Autodesk Inventor part; units mm, degrees
ref_plane "YZ Plane" through (0, 0, 0) normal (1, 0, 0) x (0, 1, 0)
ref_plane "XZ Plane" through (0, 0, 0) normal (0, 1, 0) x (-1, 0, 0)
ref_plane "XY Plane" through (0, 0, 0) normal (0, 0, 1) x (1, 0, 0)
sketch "Sketch1" plane through (0, 0, 0) normal (1, 0, 0) x (0, 1, 0)
  line L0 (0, 0) -> (0, -20)
  line L1 (0, -20) -> (8, -20)
  line L2 (8, -20) -> (3, 0)
  line L3 (3, 0) -> (0, 0)
  dimension "d0" = 8
  dimension "d1" = 20
  dimension "d11" = 3
extrude "Extrusion1" add sketch "Sketch1" along normal blind 12
sketch "Sketch2" plane through (0, 0, -20) normal (0, 0, -1) x (-1, 0, 0)
  line L0 (0, 0) -> (0, 8) construction
  line L1 (0, 8) -> (-12, 8) construction
  line L2 (-12, 0) -> (-12, 8) construction
  line L3 (0, 0) -> (-12, 0) construction
  line L4 (-12, 8) -> (0, 0) construction
  line L5 (0, 8) -> (-12, 0) construction
  point P0 (0, 0)
  point P1 (-6, 4)
hole "Hole1" at (6, 4, -20) direction (0, 0, 1) diameter 4.3 depth 7
sketch "Sketch3" plane through (0, 0, 0) normal (-1, 0, 0) x (0, 0, 1)
  line L0 (-20, 0) -> (-20, 8)
  line L1 (-20, 8) -> (0, 3)
  line L2 (0, 3) -> (0, 0)
  line L3 (0, 0) -> (-20, 0)
  line L4 (-20, 15) -> (0, 15)
  line L5 (0, 15) -> (0, 5)
  line L6 (0, 5) -> (-20, 13.9197)
  line L7 (-20, 13.9197) -> (-20, 15)
  dimension "d12" = 15
  dimension "d13" = 2
  dimension "d14" = 10
extrude "Extrusion2" add sketch "Sketch3" against normal up to surface (12 mm away) contours L4 L5 L6 L7
sketch "Sketch4" plane through (0, 0, 0) normal (-1, 0, 0) x (0, 0, 1)
  line L0 (-20, 15) -> (-20, 13.9197)
  line L1 (0, 0) -> (-20, 0)
  line L2 (-20, 15) -> (0, 15)
  line L3 (0, 15) -> (0, 0)
  line L4 (0, 0) -> (-20, 0)
  line L5 (-20, 0) -> (-20, 15)
extrude "Extrusion3" add sketch "Sketch4" along normal blind 2
sketch "Sketch5" plane through (12, 0, 0) normal (1, 0, 0) x (0, 0, -1)
  line L0 (0, 0) -> (0, 15)
  line L1 (0, 15) -> (20, 15)
  line L2 (0, 0) -> (20, 0)
  line L3 (20, 0) -> (20, 15)
  line L4 (20, 15) -> (0, 15)
  line L5 (0, 15) -> (0, 0)
extrude "Extrusion4" add sketch "Sketch5" along normal blind 2
fillet "Fillet1" radius 2 2 edges at (-2, 15, -10) (14, 15, -10)
properties part number "BeltClampNew"
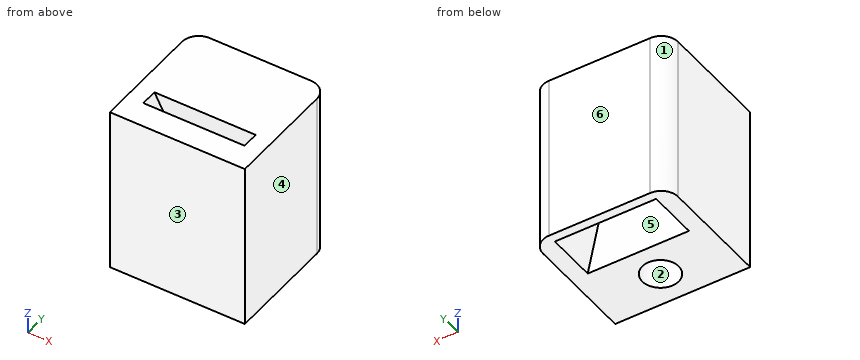
Here's how the part is built. I have some questions about the finished solid (model axes, mm). Face numbers are marked on the shaded views. A direction names the side the tool comes from. Give positions to 0.01 mm unless a question says otherwise; leave off trailing zeros. Loops run counter-clockwise (first coordinate to the right, second up) from the corner with the lowest first, then second, coordinate; pieces in that order, holes last. Notation, with made-up numbers: M 0.5,53.25 L 13.5,53.25 A22 ccw 13.5,89.25 Z; hole C 65.5,28.5 d2. An arc over 180 degrees is marked long. Return JSON: item names as keys, results as strings.
Item 1: Imagine slicing it at A-A on x = 11. List the corners of the cut face in (y, z) for me.
A:
{"outline": "M 0,-20 L 8,-20 L 3,0 L 0,0 Z; M 5,0 L 13.92,-20 L 15,-20 L 15,0 Z"}
Item 2: Please list where these lines run through material, in increasing order: line 1 (X direction, y = 8.5, z = -14); line 2 (X direction, y = 4, z = -14.75); line 3 (Y direction, x = 6, z = -15.5) (3 decimals).
A:
{"line 1": "x = -2 to 0, 12 to 14", "line 2": "x = -2 to 3.85, 8.15 to 14", "line 3": "y = 0 to 1.85, 6.15 to 6.875, 11.913 to 15"}
Item 3: I'm going to push a flat-ended pin straight in: pin 1 Ø1.5 at (x, y) = (3.5, 11) entering from -Z. Where does the tip first touch, or does it pass through?
A:
{"pin 1": "stops at z = -15.14"}
Item 4: Imagine slicing it at D-D on x = 6. List the corners of the cut face in (y, z) for me.
A:
{"outline": "M 0,-20 L 1.85,-20 L 1.85,-13 L 6.15,-13 L 6.15,-20 L 8,-20 L 3,0 L 0,0 Z; M 5,0 L 13.92,-20 L 15,-20 L 15,0 Z"}
Item 5: On a 3-axis mill with a long thin cutter (end or side, diameter ignored), from which of +Z, -Z, +X, -X, +Y, -Y can I reach the whole of each face in a straight line? I mean the marked faces 5 and 6. Say none if no direction works.
A:
{"face 5": "none", "face 6": "+Z, -Z, +X, -X, +Y"}
Item 6: Imagine slicing it at B-B on y = 4. List the corners of the cut face in (x, z) for me, then the cut area to 3 significant figures.
A:
{"outline": "M -2,-20 L 3.85,-20 L 3.85,-13 L 8.15,-13 L 8.15,-20 L 14,-20 L 14,0 L 12,0 L 12,-4 L 0,-4 L 0,0 L -2,0 Z", "area": "242 mm^2"}
Item 7: Imagine slicing it at C-C on z = -3.75. List the corners of the cut face in (x, y) for me, then the cut area to 3 significant figures.
A:
{"outline": "M -2,0 L 14,0 L 14,13 A2 ccw 12,15 L 0,15 A2 ccw -2,13 Z; hole M 0,3.94 L 12,3.94 L 12,6.67 L 0,6.67 Z", "area": "205 mm^2"}
Item 8: Thinking about a two-plate mould opening in Y: for the marked faces 1, 2, 3 and 4, which applies, released by +Y, released by -Y, zero draft, split by the parting line, or undercut?
A:
{"face 1": "released by +Y", "face 2": "undercut", "face 3": "released by -Y", "face 4": "zero draft"}
